The model under review builds one solid part; all positions refer to its coordinate system, in mm. Coordinates: 2 decimals unless noted, no trailing zeros. Write each loop counter-clockwise with the first axis right and the second up, starting at its lowest first coordinate (ties: lowest second). Pieces come first, ordered by that corner, then holes. Notation, with made-up numbers: (70, -8) - (127, -8) arc R13 ccw to (127, 12) - close; hole circle Ø6 at (-32.75, -38). An arc over 180 degrees is marked (long way). Put each result on its own line as item: value.
from build123d import *

# Parameters (mm, degrees)
SKETCH4_W           = 177.8
SKETCH4_H           = 177.8
BOSS_EXTRUDE2_DEPTH = 2.54
SKETCH5_W           = 76.2
SKETCH5_H           = 76.2
CUT_EXTRUDE1_DEPTH  = 84.074


with BuildPart() as part:
    # Sketch4 → Boss-Extrude2 (new body)
    with BuildSketch(Plane(origin=(0, 0, 0), x_dir=(1, 0, 0), z_dir=(0, 1, 0))):
        with Locations((-11.748126233, 27.003155819)):
            Rectangle(SKETCH4_W, SKETCH4_H)
    extrude(amount=-BOSS_EXTRUDE2_DEPTH)

    # Sketch5 → Cut-Extrude1 (cut)
    with BuildSketch(Plane(origin=(0, 0, 0), x_dir=(1, 0, 0), z_dir=(0, 1, 0))):
        with Locations((-11.748126233, 27.003155819)):
            Rectangle(SKETCH5_W, SKETCH5_H)
    extrude(amount=-CUT_EXTRUDE1_DEPTH, mode=Mode.SUBTRACT)


solid = part.part
1. To check wall thickness, follow probe 1 along Z at (x, y) = (5.5, -1.9); probe 2 along X at (y, z) = (-2.2, -15.5). State the ranges of each line that lie inside material, in increasing order.
Determined:
probe 1: z = -115.9 to -65.1, 11.1 to 61.9
probe 2: x = -100.65 to -49.85, 26.35 to 77.15
2. Consider section A-A on z = -11. State the section outline as (x, y) points, plus the area to 3 significant figures.
Determined:
outline: (-100.65, -2.54) - (-49.85, -2.54) - (-49.85, 0) - (-100.65, 0) - close; (26.35, -2.54) - (77.15, -2.54) - (77.15, 0) - (26.35, 0) - close
area: 258 mm^2
3. Consider section C-C on y = -0.75. State the section outline as (x, z) points, plus the area to 3 significant figures.
Determined:
outline: (-100.65, -115.9) - (77.15, -115.9) - (77.15, 61.9) - (-100.65, 61.9) - close; hole (-49.85, -65.1) - (26.35, -65.1) - (26.35, 11.1) - (-49.85, 11.1) - close
area: 25,800 mm^2
4. Consider section B-B on x = 24. State the section outline as (y, z) points, plus the area to 3 significant figures.
Determined:
outline: (-2.54, -115.9) - (0, -115.9) - (0, -65.1) - (-2.54, -65.1) - close; (-2.54, 11.1) - (0, 11.1) - (0, 61.9) - (-2.54, 61.9) - close
area: 258 mm^2
